Build history of the part. All positions in model axes, mm. A direction names the side the tool comes from. Round coordinates to 2 decimals unless told otherwise and drop trailing zeros. Loops run counter-clockwise (first coordinate to the right, second up) from the corner with the lowest first, then second, coordinate; pieces in that order, holes last. Notation, with made-up numbers: (6, 58.25) - (60, 58.25) arc R19 ccw to (60, 82.25) - close; hole circle Ø4 at (65.5, -13). An arc over 180 degrees is marked (long way). Use a Markdown table: item, result.
Solid Edge part; units mm, degrees
sketch "Sketch1" plane through (0, 0, 0) normal (0, 0, 1) x (1, 0, 0)
  circle A0 centre (0, 0) radius 17.5
extrude "Protrusion1" add sketch "Sketch1" along normal blind 180
sketch "Sketch2" plane through (0, 0, 180) normal (0, 0, 1) x (1, 0, 0)
  line L0 (-4.1, 17.0129) -> (-4.1, -17.0129)
  line L1 (4.1, 17.0129) -> (4.1, -17.0129)
  arc A0 (-4.1, 17.0129) -> (4.1, 17.0129) centre (0, 0) cw
  arc A1 (-4.1, -17.0129) -> (4.1, -17.0129) centre (0, 0) ccw
extrude "ExtrudedProtrusion_2" add sketch "Sketch2" along normal blind 25
sketch "Sketch3" plane through (4.1, 0, 212.5) normal (1, 0, 0) x (0, 1, 0)
  circle A0 centre (0, -20) radius 6.45
extrude "Cutout1" cut sketch "Sketch3" against normal up to next
sketch "Sketch4" plane through (0, 0, 0) normal (1, 0, 0) x (0, 1, 0)
  circle A0 centre (0, 20) radius 10
extrude "Cutout2" cut sketch "Sketch4" against normal through all and the other way through all
Q1. Probe line 1 (Z direction, x = 0, y = 0); line 2 (Y direction, x = -1, z = 192); line 3 (Z direction, x = -2.5, y = -4). List the from-to ranges inside material, lowest first.
Results found:
| item | result |
|---|---|
| line 1 | z = 0 to 10, 30 to 186.05, 198.95 to 205 |
| line 2 | y = -17.47 to -6.43, 6.43 to 17.47 |
| line 3 | z = 0 to 10.83, 29.17 to 187.44, 197.56 to 205 |
Q2. Cut at C-C, the plane x = 0. List the corners of the cut face in (y, z), plus the area to 3 significant figures.
Results found:
| item | result |
|---|---|
| outline | (-17.5, 0) - (17.5, 0) - (17.5, 205) - (-17.5, 205) - close; hole circle Ø20 at (0, 20); hole circle Ø12.9 at (0, 192.5) |
| area | 6,730 mm2 |
Q3. Cut at A-A, the plane y = 0. List the corners of the cut face in (x, z).
Results found:
| item | result |
|---|---|
| outline | (-17.5, 0) - (17.5, 0) - (17.5, 10) - (-17.5, 10) - close; (-17.5, 30) - (17.5, 30) - (17.5, 180) - (4.1, 180) - (4.1, 186.05) - (-4.1, 186.05) - (-4.1, 180) - (-17.5, 180) - close; (-4.1, 198.95) - (4.1, 198.95) - (4.1, 205) - (-4.1, 205) - close |
Q4. Pull direction Y, two halves, no side cores. Call faces 4 (the face through (4.1, 4, 187)), 5 (the face through (0.057, -1.398, 186.203)), 6 (the face through (-17.483, -0.769, 101.065)): pulls with the +Y half, pulls with the -Y half, needs draft (parallel to the pull), parting line crosses it, or undercut.
Results found:
| item | result |
|---|---|
| face 4 | needs draft |
| face 5 | undercut |
| face 6 | parting line crosses it |
Q5. Drop flat-ended pins along their axis: pin 1 (1 mm diameter, centred on y = -8.5, z = 99.5, fed in from -X); pin 2 (1.5 mm diameter, centred on x = -11.5, z = 163.5, fed in from +Y); pin 3 (10 mm diameter, centred on x = -9, z = 95.5, fed in from +Y). Give the stop position or say it passes through.
Results found:
| item | result |
|---|---|
| pin 1 | stops at x = -15.56 |
| pin 2 | stops at y = 13.81 |
| pin 3 | stops at y = 17.04 |
Q6. Cut at D-D, the plane x = -7.5. List the corners of the cut face in (y, z).
Results found:
| item | result |
|---|---|
| outline | (-15.81, 0) - (15.81, 0) - (15.81, 180) - (-15.81, 180) - close; hole circle Ø20 at (0, 20) |
Q7. Which spindle directions (+Z, -Z, +X, -X, +Y, -Y) get a long thin tool onto all of the face, cutting with end or side? Do faces 1 (the face through (9, 0, 180)), 2 (the face through (0, 0, 0)), 3 (the face through (-4.1, 4, 187)). Say none if no direction does.
Results found:
| item | result |
|---|---|
| face 1 | +Z, +X, +Y, -Y |
| face 2 | -Z, +X, -X, +Y, -Y |
| face 3 | +Z, -X, +Y, -Y |
Q8. Cut at B-B, the plane z = 192.5. List the corners of the cut face in (x, y), plus the area to 3 significant figures.
Results found:
| item | result |
|---|---|
| outline | (-4.1, -17.01) arc R17.5 ccw to (4.1, -17.01) - (4.1, -6.45) - (-4.1, -6.45) - close; (-4.1, 6.45) - (4.1, 6.45) - (4.1, 17.01) arc R17.5 ccw to (-4.1, 17.01) - close |
| area | 179 mm2 |
